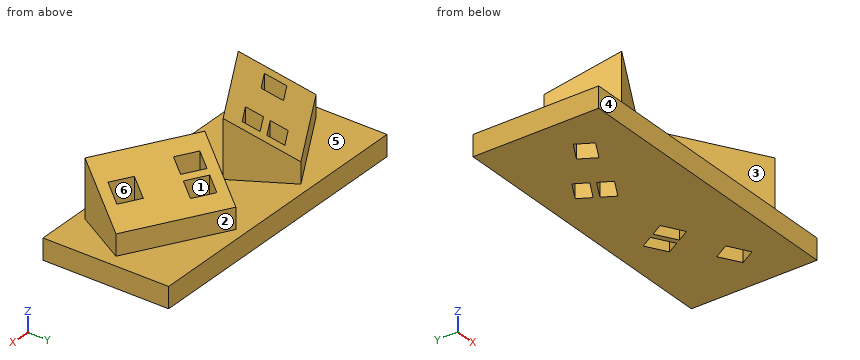
from build123d import *

# Parameters (mm, degrees)
SKETCH1_W           = 14
SKETCH1_H           = 6
BOSS_EXTRUDE1_DEPTH = 1
BOSS_EXTRUDE2_DEPTH = 10
CUT_EXTRUDE1_DEPTH  = 5
CUT_EXTRUDE4_DEPTH  = 5


with BuildPart() as part:
    # Sketch1 → Boss-Extrude1 (new body)
    with BuildSketch(Plane.XY):
        with Locations((-28.980109017, 20.469258927)):
            Rectangle(SKETCH1_W, SKETCH1_H)
    extrude(amount=BOSS_EXTRUDE1_DEPTH)

    # 3DSketch3 → Boss-Extrude2 (add)
    with BuildSketch(Plane(origin=(-35.395172526, 20.518297033, 1), x_dir=(0.9998585349462691, -0.016819931483230154, 0), z_dir=(0, 0, -1))):
        Polygon((0, 0), (4.287464629, -2.572478777), (5.830951895, 0), (1.543487266, 2.572478777), align=None)
    boss_extrude2 = extrude(amount=-BOSS_EXTRUDE2_DEPTH)

    # Sketch5 → Cut-Extrude1 (cut)
    with BuildSketch(Plane(origin=(-17.661696158, -10.196985031, 0), x_dir=(0, 0, 1), z_dir=(-0.8660254037844383, -0.5000000000000009, 0))):
        Polygon((3.732050808, 32.466952736), (11, 32.466952736), (11, 35.466952736), (2, 35.466952736), align=None)
    cut_extrude1 = extrude(amount=-CUT_EXTRUDE1_DEPTH, mode=Mode.SUBTRACT)

    # Sketch8 → Cut-Extrude4 (cut, symmetric, along a direction that is not the sketch's normal)
    with BuildSketch(Plane(origin=(-4.866381794, 8.428820516, 16.857641032), x_dir=(0.9682458365518544, 0.11180339887498851, 0.2236067977499786), z_dir=(-0.24999999999999922, 0.43301270189221724, 0.8660254037844398))):
        Polygon((-27.780523262, 17.561354254), (-26.796645351, 18.05329321), (-27.154416227, 18.768834963), (-28.138294138, 18.276896007), align=None)
        Polygon((-27.288588307, 16.577484344), (-26.304710396, 17.0694233), (-26.662481272, 17.784965053), (-27.646359183, 17.293026097), align=None)
        Polygon((-30.530878873, 16.577488345), (-30.083665278, 15.683061154), (-29.099795368, 16.174996109), (-29.547008963, 17.0694233), align=None)
    cut_extrude4 = extrude(amount=CUT_EXTRUDE4_DEPTH, dir=(0, 0, 1), both=True, mode=Mode.SUBTRACT)

    # Mirror1: Boss-Extrude2, Cut-Extrude1, Cut-Extrude4 across plane
    add(boss_extrude2.mirror(Plane.ZY.offset(28.980109017)))
    add(cut_extrude1.mirror(Plane.ZY.offset(28.980109017)), mode=Mode.SUBTRACT)
    add(cut_extrude4.mirror(Plane.ZY.offset(28.980109017)), mode=Mode.SUBTRACT)


solid = part.part
The listing builds one solid part. Answer for the finished solid, in the listing's coordinates (mm). Face numbers are marked on the shaded views. A direction names the side the tool comes from. Round coordinates to 2 decimals unless told otherwise and drop trailing zeros. Order: outer loops, then holes, each group sorted by start corner. A loop starts at its lowest first (then second) coordinate and runs counter-clockwise, first axis right, second up. Notation, with made-up numbers: (57.25, 67.5) - (101.25, 67.5) arc R12 cw to (101.25, 76.5) - close; hole circle Ø2 at (62.25, -30.75). An arc over 180 degrees is marked (long way). Write item = value, one per line. Start each with the question number.
1) For the marked faces 1, 2 and 3, determine the directions among +Z, -Z, +X, -X, +Y, -Y from which every point of the face is accessible in a straight line to the end or side of a thin tool.
2) Section A-A, the plane z = 1.45 is taken. Count the separate pieces of the cut face and the enclosed holes in it, plus the area to 3 significant figures.
3) Section B-B, the plane z = 0.25 is taken. Write down the section's boundary in (x, y).
4) Straight lines are drawn through the part: L1, parallel to X at y = 20.5, z = 0.65; L2, parallel to X at y = 19.8, z = 2.05; L3, parallel to Y at x = -26.75, z = 2.2. For each, find the intervals that lie inside material, in ascending order.
5) For a pull along Y with two mould halves and no side action, classify the marked faces 4, 5 and 6 as released by +Y, released by -Y, zero draft, split by the parting line, or undercut.
6) Section C-C, the plane y = 19.5 is taken. Write down the section's boundary in (x, z), plus the area to 3 significant figures.
7) Given pin 1 (1 mm diameter, centred on x = -34.5, z = 2, fed in from -Y), flat-ended and moving along its own axis, determine where the tip first touches the part or whether it passes through.
8) Section D-D, the plane x = -27.75 is taken. Write down the section's boundary in (y, z).
Results list:
q1.face_1 = +Z, -Z
q1.face_2 = +Z, +X, +Y
q1.face_3 = +Z, -Y
q2.separate_pieces = 2
q2.enclosed_holes = 6
q2.area = 25.0 mm^2
q3.outline = (-35.98, 17.47) - (-21.98, 17.47) - (-21.98, 23.47) - (-35.98, 23.47) - close; hole (-34.43, 19.84) - (-33.99, 19.09) - (-33.04, 19.64) - (-33.48, 20.39) - close; hole (-32.11, 21.63) - (-31.76, 21.03) - (-30.81, 21.58) - (-31.16, 22.18) - close; hole (-31.63, 20.81) - (-31.29, 20.21) - (-30.34, 20.76) - (-30.68, 21.36) - close; hole (-27.62, 20.76) - (-26.67, 20.21) - (-26.33, 20.81) - (-27.28, 21.36) - close; hole (-27.15, 21.58) - (-26.2, 21.03) - (-25.85, 21.63) - (-26.8, 22.18) - close; hole (-24.92, 19.64) - (-23.97, 19.09) - (-23.53, 19.84) - (-24.49, 20.39) - close
q4.L1 = -35.98 to -31.46, -30.78 to -27.18, -26.5 to -21.98
q4.L2 = -34.98 to -34.4, -33.13 to -30.64, -27.32 to -24.83, -23.56 to -22.98
q4.L3 = 19.47 to 20.25, 21.05 to 21.35, 22.15 to 22.53
q5.face_4 = released by -Y
q5.face_5 = zero draft
q5.face_6 = undercut
q6.outline = (-35.98, 0) - (-34.23, 0) - (-34.23, 2.85) - (-34.81, 2.68) - (-34.81, 1) - (-35.98, 1) - close; (-33.29, 0) - (-24.67, 0) - (-24.67, 3.12) - (-26.8, 3.73) - (-26.8, 1) - (-31.16, 1) - (-31.16, 3.73) - (-33.29, 3.12) - close; (-23.73, 0) - (-21.98, 0) - (-21.98, 1) - (-23.15, 1) - (-23.15, 2.68) - (-23.73, 2.85) - close
q6.area = 24.5 mm^2
q7.pin_1 = 18.1
q8.outline = (17.47, 0) - (23.47, 0) - (23.47, 1) - (21.54, 1) - (21.54, 2.99) - (20.05, 3.73) - (20.05, 1) - (17.47, 1) - close
